CAD build for the part. Positions are in the model's coordinates, mm. Face numbers are marked on the shaded views. Give positions to 0.01 mm unless a question says otherwise; leave off trailing zeros. Write each loop counter-clockwise with the first axis right and the second up, starting at its lowest first coordinate (ties: lowest second). Pieces come first, ordered by that corner, then holes. Notation, with made-up numbers: (52.25, 44.25) - (81.25, 44.25) arc R22 ccw to (81.25, 79.25) - close; hole circle Ø10 at (17, 37). An arc over 180 degrees is marked (long way). Put each result on its own line as item: value. Start each with the question number.
1. Drop flat-ended pins along their axis: pin 1 (1.5 mm diameter, centred on x = -42, y = -2, fed in from +Z); pin 2 (2.5 mm diameter, centred on y = 0, z = 47, fed in from +X); pin 3 (1.5 mm diameter, centred on x = 42, y = 0, fed in from -Z). Give the stop position or say it passes through.
2. Cut at A-A on x = 0. List the corners of the cut face in (y, z).
3. Wall check: line 1 (Z direction, x = 0, y = -2.5); line 2 (Z direction, x = -42.5, y = -0.5); line 3 (Z direction, x = -9.5, y = -4). Give the ranges that are in metal, low to high.
4. Mould opens along Z. For the marked faces 1, 2, 3 and 4 say: +Z half, -Z half, draft (parallel to the pull), parting line (faces both ways), or undercut.
5. Cut at B-B on y = -2.25. Give the number of separate pieces and of enclosed holes in the cut face, and give its area (3 significant figures).
6. Cut at C-C on z = 51.5. List the corners of the cut face in (x, y), and give its area (3 significant figures).
from build123d import *

# Parameters (mm, degrees)
F0_W           = 80
F0_H           = 120
F0_R           = 5
F0_R_2         = 2.65
F1_DEPTH       = 5
F2_W           = 80
F2_H           = 20
F3_DEPTH       = 10
F4_W           = 6
F4_H           = 6
F4_R           = 0.95
F5_DEPTH       = 10
F6_R           = 2.99999
F9_W           = 40
F9_H           = 5
F10_DEPTH      = 12
F10_DEPTH_BACK = 10


# Not quite as in the source:
# - a fillet or chamfer is up to 0.001 mm smaller than in the source, because OpenCascade refuses the exact size


with BuildPart() as f1:
    # F0 (on Front) → F1 (new body, symmetric)
    with BuildSketch(Plane.XZ):
        Rectangle(F0_W, F0_H)
        with Locations((0, 3.126)):
            Circle(F0_R, mode=Mode.SUBTRACT)
        with Locations((0, 13.126)):
            Circle(F0_R_2, mode=Mode.SUBTRACT)
    extrude(amount=F1_DEPTH, both=True)

    # F2 (on face) → F3 (cut)
    with BuildSketch(Plane.XZ.offset(5)):
        with Locations((0, -50)):
            Rectangle(F2_W, F2_H)
    extrude(amount=-F3_DEPTH, mode=Mode.SUBTRACT)

    # F4 (on face) → F5 (join)
    with BuildSketch(Plane.XZ.offset(5)):
        with Locations((43, 3)):
            Rectangle(F4_W, F4_H)
        with Locations((42.5, 3.126)):
            Circle(F4_R, mode=Mode.SUBTRACT)
    extrude(amount=-F5_DEPTH)

    # F6 (radius 3 in the source; OpenCascade refuses exactly that, so slightly less here)
    f6_edges = [f1.edges().sort_by_distance(p)[0] for p in [
        (46, 0, 0),
        (46, 0, 6),
    ]]
    fillet(f6_edges, radius=F6_R)

    # F7: F1 across plane


with BuildPart() as f1_1:
    add(f1.part)
    add(f1.part.mirror(Plane.YZ))

    # F9 (on face) → F10 (cut, two sides)
    with BuildSketch(Plane.XZ.offset(5)) as f10_sk:
        with Locations((0, 47.5)):
            Rectangle(F9_W, F9_H)
    extrude(amount=-F10_DEPTH, mode=Mode.SUBTRACT)
    extrude(f10_sk.sketch, amount=F10_DEPTH_BACK, mode=Mode.SUBTRACT)


solid = f1_1.part
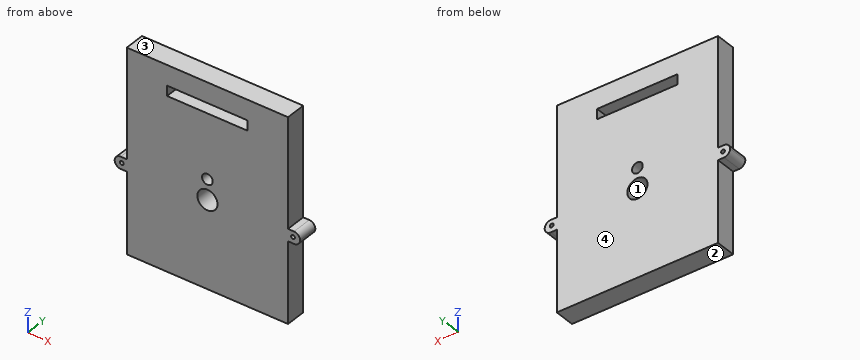
Report:
1. pin 1: stops at z = 6
1. pin 2: stops at x = 40
1. pin 3: stops at z = 0
2. outline: (-5, -40) - (5, -40) - (5, -1.87) - (-5, -1.87) - close; (-5, 8.13) - (5, 8.13) - (5, 10.48) - (-5, 10.48) - close; (-5, 15.78) - (5, 15.78) - (5, 45) - (-5, 45) - close; (-5, 50) - (5, 50) - (5, 60) - (-5, 60) - close
3. line 1: z = -40 to -1.87, 8.13 to 10.48, 15.78 to 45, 50 to 60
3. line 2: z = 0 to 2.18, 4.08 to 6
3. line 3: z = -40 to 45, 50 to 60
4. face 1: undercut
4. face 2: -Z half
4. face 3: +Z half
4. face 4: draft
5. separate pieces: 1
5. enclosed holes: 5
5. area: 7,760 mm²
6. outline: (-40, -5) - (40, -5) - (40, 5) - (-40, 5) - close
6. area: 800 mm²
